Check sheet for the modelled part. Datum: model origin and axes. Units: mm. A direction names the side the tool comes from. Round coordinates to 2 decimals unless told otherwise and drop trailing zeros. Write each loop counter-clockwise with the first axis right and the second up, starting at its lowest first coordinate (ties: lowest second). Pieces come first, ordered by that corner, then holes. Notation, with made-up numbers: M 37,31.5 L 46,31.5 A22 ccw 46,50.5 Z; hole C 30,48 d3. An arc over 180 degrees is marked long. One line per item, written item: value.
Autodesk Inventor part; units mm, degrees
ref_plane "YZ Plane" through (0, 0, 0) normal (1, 0, 0) x (0, 1, 0)
ref_plane "XZ Plane" through (0, 0, 0) normal (0, 1, 0) x (-1, 0, 0)
ref_plane "XY Plane" through (0, 0, 0) normal (0, 0, 1) x (1, 0, 0)
sketch "Esboço1" plane through (0, 0, 0) normal (0, 0, 1) x (1, 0, 0)
  line L0 (-29.6595, 42.7148) -> (-29.6595, -23.7852) construction
  line L1 (-29.6595, 42.7148) -> (65.3405, 42.7148) construction
  line L2 (65.3405, 42.7148) -> (65.3405, -23.7852) construction
  line L3 (65.3405, -23.7852) -> (-29.6595, -23.7852) construction
  circle A0 centre (65.3405, 42.7148) radius 2.5
  circle A1 centre (65.3405, -23.7852) radius 2.5
  circle A2 centre (-29.6595, 42.7148) radius 2.5
  circle A3 centre (-29.6595, -23.7852) radius 2.5
  line L4 (65.3405, 42.7148) -> (65.3405, 46.7148) construction
  line L5 (65.3405, 46.7148) -> (-29.6595, 46.7148) construction
  line L6 (-29.6595, 46.7148) -> (-29.6595, 42.7148) construction
  line L7 (65.3405, -23.7852) -> (65.3405, -27.7852) construction
  line L8 (65.3405, -27.7852) -> (-29.6595, -27.7852) construction
  line L9 (-29.6595, -27.7852) -> (-29.6595, -23.7852) construction
  line L10 (17.8405, 42.7148) -> (-37.1595, 42.7148) construction
  line L11 (17.8405, 42.7148) -> (72.8405, 42.7148) construction
  line L12 (17.8405, -23.7852) -> (-47.1595, -23.7852) construction
  line L13 (17.8405, -23.7852) -> (62.8405, -23.7852) construction
  line L14 (-29.6595, 46.7148) -> (-69.6595, 46.7148) construction
  line L15 (65.3405, -27.7852) -> (105.3405, -27.7852) construction
  line L16 (-39.6595, 46.7148) -> (75.3405, 46.7148)
  line L17 (105.3405, 16.7148) -> (105.3405, 2.2148)
  line L18 (75.3405, -27.7852) -> (-39.6595, -27.7852)
  line L19 (-69.6595, 2.2148) -> (-69.6595, 16.7148)
  arc A4 (-39.6595, 46.7148) -> (-69.6595, 16.7148) centre (-39.6595, 16.7148) ccw
  arc A5 (-69.6595, 2.2148) -> (-39.6595, -27.7852) centre (-39.6595, 2.2148) ccw
  arc A6 (105.3405, 16.7148) -> (75.3405, 46.7148) centre (75.3405, 16.7148) ccw
  arc A7 (75.3405, -27.7852) -> (105.3405, 2.2148) centre (75.3405, 2.2148) ccw
  dimension "d16" = 66.5
  dimension "d19" = 5
  dimension "d20" = 4
  dimension "d21" = 4
  dimension "d22" = 55
  dimension "d23" = 55
  dimension "d24" = 40
  dimension "d25" = 40
  dimension "d26" = 30
  dimension "d27" = 30
extrude "Extrusão1" add sketch "Esboço1" along normal blind 5
sketch "Esboço2" plane through (0, 0, 5) normal (0, 0, 1) x (1, 0, 0)
  circle A0 centre (-29.6595, 42.7148) radius 2.5 construction
  line L0 (-29.6595, 40.2148) -> (-29.6595, 36.2148) construction
  circle A1 centre (65.3405, -23.7852) radius 2.5 construction
  line L1 (65.3405, -21.2852) -> (65.3405, -17.2852) construction
  line L2 (-29.6595, 36.2148) -> (-29.6595, 36.2148) construction
  line L3 (65.3405, -17.2852) -> (65.3405, -17.2852) construction
  line L4 (85.3405, 16.2148) -> (85.3405, 2.7148)
  line L5 (-49.6595, 2.7148) -> (-49.6595, 16.2148)
  arc A2 (-29.6595, 36.2148) -> (-49.6595, 16.2148) centre (-29.6595, 16.2148) ccw
  arc A3 (-49.6595, 2.7148) -> (-29.6595, -17.2852) centre (-29.6595, 2.7148) ccw
  arc A4 (85.3405, 16.2148) -> (65.3405, 36.2148) centre (65.3405, 16.2148) ccw
  arc A5 (65.3405, -17.2852) -> (85.3405, 2.7148) centre (65.3405, 2.7148) ccw
  line L6 (65.3405, 36.2148) -> (-29.6595, 36.2148)
  line L7 (-29.6595, -17.2852) -> (65.3405, -17.2852)
  point P0 (0, 0)
  dimension "d34" = 20
extrude "Extrusão2" add sketch "Esboço2" along normal blind 5
sketch "Esboço3" plane through (0, 0, 0) normal (0, 0, -1) x (-1, 0, 0)
  circle A0 centre (-16.9737, 8.0827) radius 16.0131
  circle A1 centre (-16.9737, 8.0827) radius 11.1486
  point P0 (0, 0)
extrude "Extrusão3" add sketch "Esboço3" along normal blind 10
sketch "Esboço4" plane through (16.9737, 8.0827, -10) normal (0, 0, -1) x (-1, 0, 0)
  circle A0 centre (-6.1571, -0.3724) radius 2
  circle A1 centre (6.017, -0.3724) radius 2
  point P0 (16.9737, -8.0827)
  dimension "d39" = 4
sketch "Esboço5" plane through (16.9737, 8.0827, -10) normal (0, 0, -1) x (-1, 0, 0)
  circle A0 centre (-6.1295, -0.4053) radius 1.2064
  circle A1 centre (5.9792, -0.4053) radius 1.3709
  point P0 (16.9737, -8.0827)
extrude "Extrusão4" add sketch "Esboço4" against normal blind 10
hole "Furo1" at (23.1031, 7.6774, -10) at (10.9944, 7.6774, -10) direction (0, 0, 1) diameter 3 depth 3 tip angle 118
sketch "Esboço6" plane through (10.9567, 7.7102, -10) normal (0, 0, -1) x (-1, 0, 0)
  circle A0 centre (0, 0) radius 2
sketch "Esboço7" plane through (23.1307, 7.7102, -10) normal (0, 0, -1) x (-1, 0, 0)
  circle A0 centre (0, 0) radius 2
properties part number "luz de freio"
Q1. Draft check along Y on faces 4 (the cylindrical face through (96.79, -18.76, 2.46)), 5 (the cylindrical face through (10.544, 9.108, -8.479)), 6 (the flat face through (17, -23, 5)), 7 (the cylindrical face through (67.725, 41.964, 2.465)). Enter one of: pulls with the +Y half, pulls with the -Y half, needs draft (parallel to the pull), parting line crosses it, or undercut.
Completed:
face 4: pulls with the -Y half
face 5: undercut
face 6: needs draft
face 7: undercut
Q2. Scan lines: line 1 (Z direction, x = 80.5, y = -23.5); line 2 (Z direction, x = 4.5, y = 24); line 3 (X direction, y = 18, z = 4). Record each from-to range of solid material in increasing order. Write a range as [from, to].
Completed:
line 1: [0, 5]
line 2: [0, 10]
line 3: [-69.63, 105.31]
Q3. Sectioned sample at B-B on x = -8.5. Enter the section's corners in (y, z).
Completed:
outline: M -27.79,0 L 46.71,0 L 46.71,5 L 36.21,5 L 36.21,10 L -17.29,10 L -17.29,5 L -27.79,5 Z
Q4. Sectioned sample at C-C on y = 27. Enter the section's corners in (x, z).
Completed:
outline: M -67.84,0 L 103.52,0 L 103.52,5 L 82.18,5 L 82.18,10 L -46.5,10 L -46.5,5 L -67.84,5 Z
Q5. Access from +Z, -Z, +X, -X, +Y, -Y to the whole of each face (thin tool, end or side, straight path). Record for faces 1 (the flat face through (85.34, 10, 7)), 2 (the cylindrical face through (79.64, -11.27, 7.46)), 3 (the cylindrical face through (24.434, 8.37, -8.479)).
Completed:
face 1: +Z, +X, +Y, -Y
face 2: +Z, +X, -Y
face 3: -Z
Q6. Sectioned sample at D-D on x = -57.5. Enter the section's corners in (y, z), and give its area (3 significant figures).
Completed:
outline: M -21.9,0 L 40.83,0 L 40.83,5 L -21.9,5 Z
area: 314 mm^2
Q7. Sectioned sample at A-A on z = 1.75. Enter the section's corners in (x, y), and give its area (3 significant figures).
Completed:
outline: M -69.66,2.21 A30 ccw -39.66,-27.79 L 75.34,-27.79 A30 ccw 105.34,2.21 L 105.34,16.71 A30 ccw 75.34,46.71 L -39.66,46.71 A30 ccw -69.66,16.71 Z; hole C -29.66,-23.79 d5; hole C -29.66,42.71 d5; hole C 65.34,-23.79 d5; hole C 65.34,42.71 d5
area: 12,200 mm^2
Q8. Depth check by flat-ended pin: P1, Ø2.5, axis at x = 35, z = 7.5, coming from the +Y side; P2, Ø24.5, axis at x = 17, y = 12.5, coming from the -Z side; P3, Ø3, axis at y = 34, z = 4, coming from the -X side; P4, Ø2.5, axis at x = 23.1, y = 7.68, coming from the -Z side. Enter the tip coordinate at first touch or a pass-through.
Completed:
P1: y = 36.21
P2: z = -10
P3: x = -65.17
P4: z = -6.85
